from build123d import *

# Parameters (mm, degrees)
SKETCH_1_R          = 10
SKETCH_1_R_2        = 2.65
EXTRUDE_1_DEPTH     = 4.5
SKETCH_2_W          = 20
SKETCH_2_H          = 4.5
EXTRUDE_2_DEPTH     = 17
SKETCH_3_R          = 2.65
CUT_EXTRUDE_1_DEPTH = 17
CHAMFER_1_SIZE      = 2.65


with BuildPart() as part:
    # 草图1 → 凸台-拉伸1 (new body)
    # profile 1 of 3: a face of its own
    with BuildSketch(Plane(origin=(0, 0, 0), x_dir=(1, 0, 0), z_dir=(0, 1, 0))):
        with BuildLine():
            Line((0, 10), (-10, 10))
            Line((-10, 10), (-10, 0))
            ThreePointArc((-10, 0), (-7.071067812, 7.071067812), (0, 10))
        make_face()
    # profile 2 of 3: a face of its own
    with BuildSketch(Plane(origin=(0, 0, 0), x_dir=(1, 0, 0), z_dir=(0, 1, 0))):
        with BuildLine():
            Line((10, 10), (0, 10))
            ThreePointArc((0, 10), (7.071067812, 7.071067812), (10, 0))
            Line((10, 0), (10, 10))
        make_face()
    # profile 3 of 3: a face of its own
    with BuildSketch(Plane(origin=(0, 0, 0), x_dir=(1, 0, 0), z_dir=(0, 1, 0))):
        Circle(SKETCH_1_R)
        with Locations(Location((0, 0, 0), (0, 0, 270))):
            Circle(SKETCH_1_R_2, mode=Mode.SUBTRACT)
    extrude(amount=EXTRUDE_1_DEPTH)

    # 草图2 → 凸台-拉伸2 (add)
    with BuildSketch(Plane(origin=(0, 4.5, 0), x_dir=(1, 0, 0), z_dir=(0, 1, 0))):
        with Locations((0, 7.75)):
            Rectangle(SKETCH_2_W, SKETCH_2_H)
    extrude(amount=EXTRUDE_2_DEPTH)

    # 草图3 → 切除-拉伸1 (cut)
    with BuildSketch(Plane.XY.offset(-5.5)):
        with Locations((0, 13)):
            Circle(SKETCH_3_R)
    extrude(amount=-CUT_EXTRUDE_1_DEPTH, mode=Mode.SUBTRACT)

    # 倒角1
    chamfer_1_edges = [part.edges().sort_by_distance(p)[0] for p in [
        (0, 4.5, -2.65),
        (-2.65, 13, -5.5),
    ]]
    chamfer(chamfer_1_edges, length=CHAMFER_1_SIZE)


solid = part.part
Geometry: final body of the model. Coordinates: model frame, mm. A direction names the side the tool comes from. Give positions to 0.01 mm unless a question says otherwise; leave off trailing zeros. Loops run counter-clockwise (first coordinate to the right, second up) from the corner with the lowest first, then second, coordinate; pieces in that order, holes last. Notation, with made-up numbers: M -31,84 L -22,84 A19 cw -22,109 Z; hole C 44.25,24 d2. An arc over 180 degrees is marked long. Put each result on its own line as item: value.
1) First-contact query: P1, Ø12, axis at x = -6.5, z = -1.5, coming from the +Y side; P2, Ø7, axis at x = 0, y = 13, coming from the +Z side. Flat tips, straight axial feed; report the tip coordinate or a pass-through.
Computed values:
P1: stops at y = 21.5
P2: stops at z = -7.3
2) Reachability of faces 1 (the flat face through (0, 21.5, -8)), 2 (the flat face through (0, 19, -5.5)) from +Z, -Z, +X, -X, +Y, -Y: full face, straight path, thin tool, end or side. Return the list, or none.
Computed values:
face 1: +Z, -Z, +X, -X, +Y
face 2: +Z, +X, -X, +Y
3) Cut plane C-C, the plane z = -7.75. Return the cut outline in (x, y), plus the area to 3 significant figures.
Computed values:
outline: M -10,0 L 10,0 L 10,21.5 L -10,21.5 Z; hole C 0,13 d6.1
area: 401 mm^2
4) Cut plane A-A, the plane x = 0. Return the cut outline in (y, z).
Computed values:
outline: M 0,-10 L 10.35,-10 L 10.35,-8.15 L 7.7,-5.5 L 4.5,-5.5 L 4.5,-5.3 L 1.85,-2.65 L 0,-2.65 Z; M 0,2.65 L 1.85,2.65 L 4.5,5.3 L 4.5,10 L 0,10 Z; M 15.65,-10 L 21.5,-10 L 21.5,-5.5 L 18.3,-5.5 L 15.65,-8.15 Z
5) Cut plane B-B, the plane y = 13. Return the cut outline in (x, z), plus the area to 3 significant figures.
Computed values:
outline: M -10,-10 L -2.65,-10 L -2.65,-8.15 L -5.3,-5.5 L -10,-5.5 Z; M 2.65,-10 L 10,-10 L 10,-5.5 L 5.3,-5.5 L 2.65,-8.15 Z
area: 59.1 mm^2
6) Cut plane D-D, the plane y = 4. Return the cut outline in (x, z).
Computed values:
outline: M -10,-10 L 10,-10 L 10,0 A10 ccw -10,0 Z; hole C 0,0 d9.6
7) Mould query, pull axis Y, two halves, no side actions, for faces 3 (the flat face through (2, 0, -2)), 4 (the cylindrical face through (1.223, 10.649, -9.062)), 5 (the conical face through (-1.06, 1.98, 2.57)). Classes: released by +Y, released by -Y, zero draft, split by the parting line, or undercut.
Computed values:
face 3: released by -Y
face 4: undercut
face 5: released by +Y
8) Material intervals for L1, parallel to Y at x = 0, z = -9.3; L2, parallel to Z at x = 9, y = 9.75; L3, parallel to Y at x = -6, z = 4.5, sorted ascending. Write a range as from..to.
Computed values:
L1: y = 0..10.35, 15.65..21.5
L2: z = -10..-5.5
L3: y = 0..4.5
